Could you check a few things on this model? Use its own coordinates, in mm. Face numbers are marked on the shaded views. A direction names the side the tool comes from. Round coordinates to 2 decimals unless told otherwise and drop trailing zeros. Loops run counter-clockwise (first coordinate to the right, second up) from the corner with the lowest first, then second, coordinate; pieces in that order, holes last. Notation, with made-up numbers: (-24.75, -35) -> (15.25, -35) arc R14 cw to (15.25, -25) -> close; hole circle Ø8 at (-32.75, 74.5). An arc over 180 degrees is marked (long way). Write each question's results on one line, items separated by ' | '. Start each with the question number.
1) We'd pull the mould along Z, two halves only. Please class the marked faces 4, 5, 6 and 7: pulls with the +Z half, pulls with the -Z half, needs draft (parallel to the pull), parting line crosses it, or undercut.
2) Imagine slicing it at A-A, the plane z = -10.5. List the corners of the cut face in (x, y) for me, plus the area to 3 significant figures.
3) For P1, Ø5.5, axis at x = 16.4, y = 32.5, coming from the +Z side; P2, Ø2, axis at y = 13.5, z = -1.5, coming from the -X side; P3, Ø8, axis at x = 14.5, y = 29, coming from the +Z side; P4, Ø2.5, axis at x = 16.4, y = 6.5, coming from the -Z side, each with a flat end and sliding along its axis, tell me the tip position at first contact or that it passes through.
4) Imagine slicing it at C-C, the plane z = -22. List the corners of the cut face in (x, y) for me, plus the area to 3 significant figures.
5) Imagine slicing it at B-B, the plane y = 6.5. List the corners of the cut face in (x, z) for me, plus the area to 3 significant figures.
6) Which directions (+Z, -Z, +X, -X, +Y, -Y) give clear straight access to the entire face, cutting with the end or side of a thin tool? Please do the marked faces 1, 2 and 3.
7) Imagine slicing it at D-D, the plane z = -16. List the corners of the cut face in (x, y) for me, plus the area to 3 significant figures.
8) If I drill on probe 1 along X at (y, z) = (7.5, -27); probe 2 along X at (y, z) = (33, -26.5); probe 3 along Y at (x, z) = (-16, -24.5), over which ranges is the centre line in solid material (lowest first)?
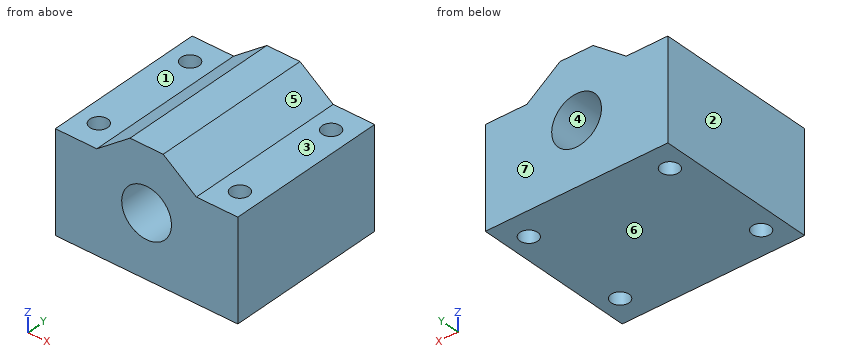
from build123d import *

# Parameters (mm, degrees)
SKETCH1_R           = 6
BOSS_EXTRUDE1_DEPTH = 39
SKETCH2_R           = 2.15
CUT_EXTRUDE1_DEPTH  = 52.06627412


with BuildPart() as part:
    # Sketch1 → Boss-Extrude1 (new body)
    with BuildSketch(Plane(origin=(0, 0, 0), x_dir=(1, 0, 0), z_dir=(0, 1, 0))):
        Polygon((21.399903705, 28.649644043), (-22.600096295, 28.649644043), (-22.600096295, 4.649644043), (-12.600096295, 4.649644043), (-4.600096295, -1.350355957), (3.399903705, -1.350355957), (11.399903705, 4.649644043), (21.399903705, 4.649644043), align=None)
        with Locations(Location((-0.600096295, 13.649644043, 0), (0, 0, 270))):
            Circle(SKETCH1_R, mode=Mode.SUBTRACT)
    extrude(amount=BOSS_EXTRUDE1_DEPTH)

    # Sketch2 → Cut-Extrude1 (cut, through all)
    with BuildSketch(Plane.XY.offset(-4.649644043)):
        with Locations((-17.600096295, 32.5)):
            Circle(SKETCH2_R)
        with Locations((-17.600096295, 6.5)):
            Circle(SKETCH2_R)
        with Locations(Location((16.399903705, 6.5, 0), (0, 0, 180))):
            Circle(SKETCH2_R)
        with Locations(Location((16.399903705, 32.5, 0), (0, 0, 180))):
            Circle(SKETCH2_R)
    extrude(amount=-CUT_EXTRUDE1_DEPTH, mode=Mode.SUBTRACT)


solid = part.part
Checked values:
1) face 4: undercut | face 5: pulls with the +Z half | face 6: pulls with the -Z half | face 7: needs draft
2) outline: (-22.6, 0) -> (-5.71, 0) -> (-5.71, 39) -> (-22.6, 39) -> close; (4.51, 0) -> (21.4, 0) -> (21.4, 39) -> (4.51, 39) -> close; hole circle Ø4.3 at (-17.6, 6.5); hole circle Ø4.3 at (-17.6, 32.5); hole circle Ø4.3 at (16.4, 6.5); hole circle Ø4.3 at (16.4, 32.5) | area: 1,260 mm^2
3) P1: z = -4.65 | P2: x = -9.73 | P3: z = -3.97 | P4: through
4) outline: (-22.6, 0) -> (21.4, 0) -> (21.4, 39) -> (-22.6, 39) -> close; hole circle Ø4.3 at (-17.6, 6.5); hole circle Ø4.3 at (-17.6, 32.5); hole circle Ø4.3 at (16.4, 6.5); hole circle Ø4.3 at (16.4, 32.5) | area: 1,660 mm^2
5) outline: (-22.6, -28.65) -> (-19.75, -28.65) -> (-19.75, -4.65) -> (-22.6, -4.65) -> close; (-15.45, -28.65) -> (14.25, -28.65) -> (14.25, -4.65) -> (11.4, -4.65) -> (3.4, 1.35) -> (-4.6, 1.35) -> (-12.6, -4.65) -> (-15.45, -4.65) -> close; (18.55, -28.65) -> (21.4, -28.65) -> (21.4, -4.65) -> (18.55, -4.65) -> close; hole circle Ø12 at (-0.6, -13.65) | area: 833 mm^2
6) face 1: +Z, -X, +Y, -Y | face 2: +Z, -Z, -X, +Y, -Y | face 3: +Z, +X, +Y, -Y
7) outline: (-22.6, 0) -> (-6.12, 0) -> (-6.12, 39) -> (-22.6, 39) -> close; (4.92, 0) -> (21.4, 0) -> (21.4, 39) -> (4.92, 39) -> close; hole circle Ø4.3 at (-17.6, 6.5); hole circle Ø4.3 at (-17.6, 32.5); hole circle Ø4.3 at (16.4, 6.5); hole circle Ø4.3 at (16.4, 32.5) | area: 1,230 mm^2
8) probe 1: -22.6 to -19.5, -15.7 to 14.5, 18.3 to 21.4 | probe 2: -22.6 to -19.69, -15.51 to 14.31, 18.49 to 21.4 | probe 3: 0 to 5.06, 7.94 to 31.06, 33.94 to 39
